Verification items for the finished model (mm, model axes). Coordinates: 2 decimals unless noted, no trailing zeros. Loops run counter-clockwise (first coordinate to the right, second up) from the corner with the lowest first, then second, coordinate; pieces in that order, holes last. Notation, with made-up numbers: (-33, -28) - (11, -28) arc R13 cw to (11, -5) - close; hole circle Ø10 at (-28, 42). An arc over 180 degrees is marked (long way). Answer as CSV lines item,"result". Start each with the question number.
1. Cross-section at B-B (x = -5). Enter the section's corners in (y, z), plus the area to 3 significant figures.
2. Cross-section at A-A (y = 0.1). Enter the section's corners in (x, z).
3. Material ranges on line 1 (Z direction, x = -1.5, y = 0.05); line 2 (Z direction, x = 15, y = 0.05), recorded low to high. Write a range as [from, to].
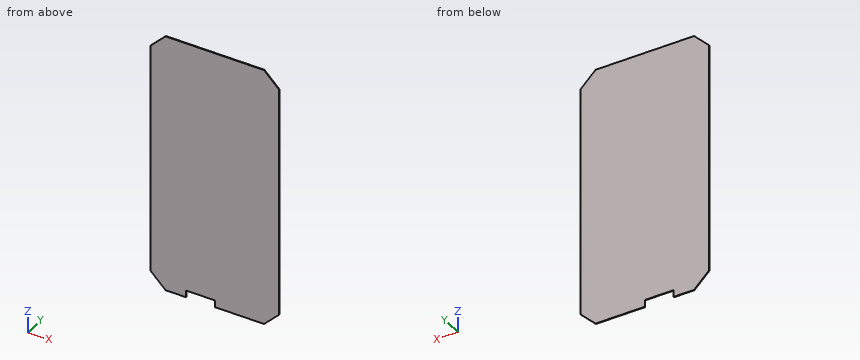
```python
from build123d import *

# Parameters (mm, degrees)
SKETCH1_W           = 34
SKETCH1_H           = 69.8
BOSS_EXTRUDE1_DEPTH = 0.18
CHAMFER1_SIZE       = 4
SKETCH2_W           = 7.6
SKETCH2_H           = 1.85
CUT_EXTRUDE1_DEPTH  = 1.18


with BuildPart() as part:
    # Sketch1 → Boss-Extrude1 (new body)
    with BuildSketch(Plane(origin=(0, 0, 0), x_dir=(1, 0, 0), z_dir=(0, 1, 0))):
        Rectangle(SKETCH1_W, SKETCH1_H)
    extrude(amount=BOSS_EXTRUDE1_DEPTH)

    # Chamfer1
    chamfer1_edges = [part.edges().sort_by_distance(p)[0] for p in [
        (17, 0.09, 34.9),
        (-17, 0.09, 34.9),
        (-17, 0.09, -34.9),
        (17, 0.09, -34.9),
    ]]
    chamfer(chamfer1_edges, length=CHAMFER1_SIZE)

    # Sketch2 → Cut-Extrude1 (cut, through all)
    with BuildSketch(Plane(origin=(0, 0.18, 0), x_dir=(1, 0, 0), z_dir=(0, 1, 0))):
        with Locations((-3.8, 33.975)):
            Rectangle(SKETCH2_W, SKETCH2_H)
    extrude(amount=-CUT_EXTRUDE1_DEPTH, mode=Mode.SUBTRACT)


solid = part.part
```
Values follow:
1,outline,"(0, -33.05) - (0.18, -33.05) - (0.18, 34.9) - (0, 34.9) - close"
1,area,"12.2 mm²"
2,outline,"(-17, -30.9) - (-13, -34.9) - (-7.6, -34.9) - (-7.6, -33.05) - (0, -33.05) - (0, -34.9) - (13, -34.9) - (17, -30.9) - (17, 30.9) - (13, 34.9) - (-13, 34.9) - (-17, 30.9) - close"
3,line 1,"z = [-33.05, 34.9]"
3,line 2,"z = [-32.9, 32.9]"
